Build history of the part. All positions in model axes, mm. A direction names the side the tool comes from. Round coordinates to 2 decimals unless told otherwise and drop trailing zeros. Order: outer loops, then holes, each group sorted by start corner. A loop starts at its lowest first (then second) coordinate and runs counter-clockwise, first axis right, second up. Notation, with made-up numbers: (82, 16.5) - (110, 16.5) arc R33 cw to (110, 54.5) - close; hole circle Ø2 at (88, 48). An arc over 180 degrees is marked (long way). Write each question's results on one line, items separated by ' | '. Start each with the question number.
```python
from build123d import *

# Parameters (mm, degrees)
F0_R     = 97
F0_R_2   = 29.25
F1_DEPTH = 2
F0_R_3   = 100
F2_DEPTH = 20
F0_R_4   = 26.25
F3_DEPTH = 80
F5_R     = 27.25
F6_DEPTH = 3
F7_R     = 1.1
F8_SIZE  = 1


with BuildPart() as f1:
    # F0 (on Top) → F1 (new body)
    with BuildSketch(Plane.XY):
        Circle(F0_R)
        Circle(F0_R_2, mode=Mode.SUBTRACT)
    extrude(amount=F1_DEPTH)

    # F0 (on Top) → F2 (join)
    with BuildSketch(Plane.XY):
        Circle(F0_R_3)
        Circle(F0_R, mode=Mode.SUBTRACT)
    extrude(amount=F2_DEPTH)

    # F0 (on Top) → F3 (join)
    with BuildSketch(Plane.XY):
        Circle(F0_R_2)
        Circle(F0_R_4, mode=Mode.SUBTRACT)
    extrude(amount=F3_DEPTH)

    # F5 (on offset) → F6 (join)
    with BuildSketch(Plane.XY.offset(20)):
        Circle(F5_R)
    extrude(amount=F6_DEPTH)

    # F7
    f7_edges = [f1.edges().sort_by_distance(p)[0] for p in [
        (-100, 0, 20),
        (-97, 0, 20),
        (-29.25, 0, 80),
        (-26.25, 0, 80),
    ]]
    fillet(f7_edges, radius=F7_R)

    # F8
    f8_edges = [f1.edges().sort_by_distance(p)[0] for p in [
        (-26.25, 0, 0),
    ]]
    chamfer(f8_edges, length=F8_SIZE)


solid = f1.part
```
1. Flat gauge pins, fed straight in: pin 1 Ø5 at (x, z) = (53.5, 19) entering from +Y; pin 2 Ø16 at (x, y) = (-3, 4.5) entering from -Z; pin 3 Ø1 at (y, z) = (3.5, 51.5) entering from -X. Where does each tip first touch, or does it go through?
2. Mould opens along X. For faces 4 (the face through (44.76, -86.056, 10.332)), 5 (the face through (-4.3, 27.2, 80)), 6 (the face through (95.38, 30.04, 9.32)) say: pulls with the +X half, pulls with the -X half, needs draft (parallel to the pull), parting line crosses it, or undercut.
3. Cut at D-D (z = 59.5). List the corners of the cut face in (x, y), plus the area to 3 significant figures.
4. 3-axis set-ups, long thin cutter, end or side, ignore diameter. For faces 1 (the face through (21, -21, 0)), 2 (the face through (25, 8, 10)), 3 (the face through (25, 8, 51)): which of +Z, -Z, +X, -X, +Y, -Y reach the whole face in a straight line?
5. Wall check: line 1 (Y direction, x = 0, z = 7); line 2 (Y direction, x = 0, z = 59); line 3 (Z direction, x = 54, y = 30). Give the ranges that are in metal, low to high. Write a range as from..to.
6. Cut at B-B (z = 11.5). List the corners of the cut face in (x, y).
A:
1) pin 1: stops at y = 86.02 | pin 2: stops at z = 20 | pin 3: stops at x = -29.1
2) face 4: undercut | face 5: needs draft | face 6: parting line crosses it
3) outline: circle Ø58.5 at (0, 0); hole circle Ø52.5 at (0, 0) | area: 523 mm^2
4) face 1: -Z, +X, -X, +Y, -Y | face 2: -Z | face 3: +Z
5) line 1: y = -100..-97, -29.25..-26.25, 26.25..29.25, 97..100 | line 2: y = -29.25..-26.25, 26.25..29.25 | line 3: z = 0..2
6) outline: circle Ø200 at (0, 0); circle Ø58.5 at (0, 0); hole circle Ø194 at (0, 0); hole circle Ø52.5 at (0, 0)
